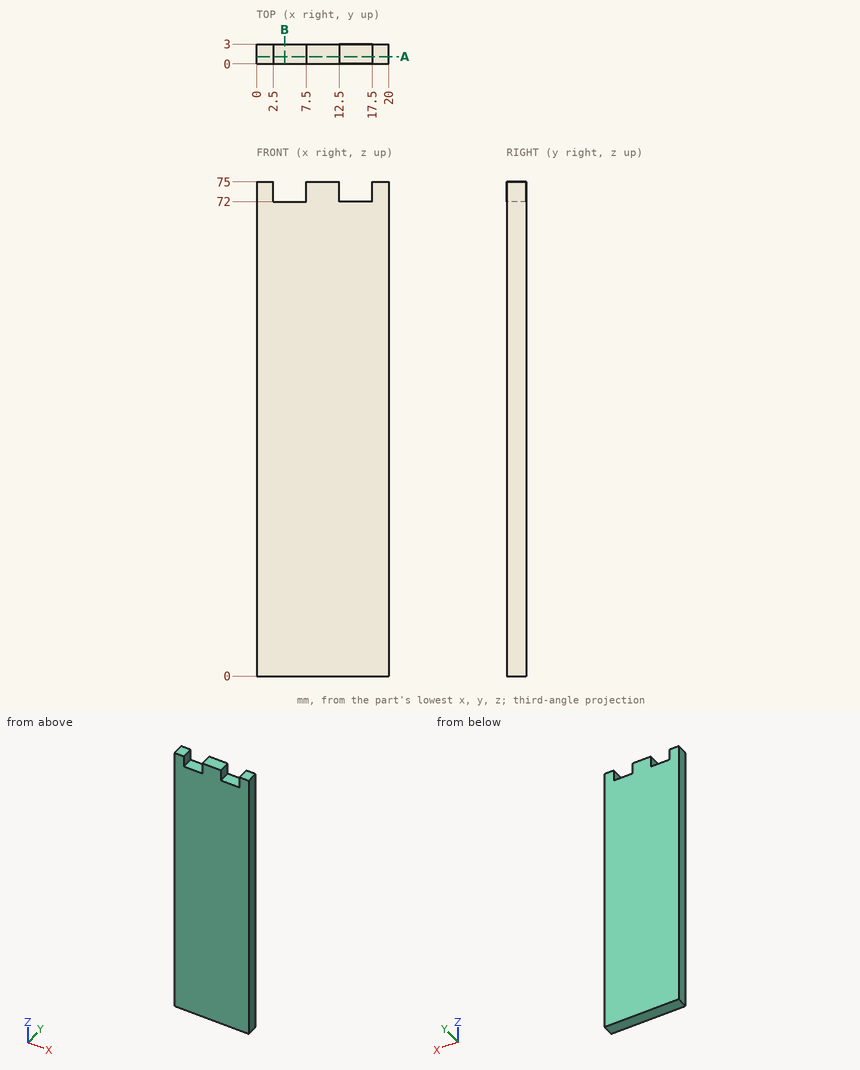
The drawing under review shows one solid part. Ordinate dimensions are in mm from its lowest x, y, z. Coordinates: 2 decimals unless noted, no trailing zeros. Order: outer loops, then holes, each group sorted by start corner. A loop starts at its lowest first (then second) coordinate and runs counter-clockwise, first axis right, second up. Notation, with made-up numbers: (10, 66) -> (29, 66) arc R16 cw to (29, 78) -> close; hole circle Ø1 at (-7.75, -26). An arc over 180 degrees is marked (long way). Answer as CSV lines item,"result".
Q1. Clearance check with a flat-ended pin moving along its axis: pin 1 Ø0.9 at (x, y) = (6, 2) entering from +Z. State where the tip first meets the part, or that it passes through.
Model answer:
pin 1,"stops at z = 72"
Q2. Wall thickness on line 1 along Z through (x, y) = (6.5, 2.05): over which ranges is the line inside the solid? List them lowest first. Write a range as [from, to].
Model answer:
line 1,"z = [0, 72]"
Q3. We need section A-A (y = 1.1). State the section outline as (x, z) points.
Model answer:
outline,"(0, 0) -> (20, 0) -> (20, 75) -> (17.5, 75) -> (17.5, 72) -> (12.5, 72) -> (12.5, 75) -> (7.5, 75) -> (7.5, 72) -> (2.5, 72) -> (2.5, 75) -> (0, 75) -> close"
Q4. We need section B-B (x = 4.25). State the section outline as (y, z) points, plus the area to 3 significant figures.
Model answer:
outline,"(0, 0) -> (3, 0) -> (3, 72) -> (0, 72) -> close"
area,"216 mm2"
